from build123d import *

# Parameters (mm, degrees)
SKETCH1_W           = 40
SKETCH1_H           = 43
SKETCH1_R           = 1.5
SKETCH1_R_2         = 5
BOSS_EXTRUDE1_DEPTH = 3
SKETCH3_R           = 1.6
BOSS_EXTRUDE2_DEPTH = 3
FILLET1_R           = 2


with BuildPart() as part:
    # Sketch1 → Boss-Extrude1 (new body)
    with BuildSketch(Plane(origin=(0, 0, 0), x_dir=(1, 0, 0), z_dir=(0, 1, 0))):
        Rectangle(SKETCH1_W, SKETCH1_H)
        with Locations((-15, -11.5)):
            Circle(SKETCH1_R, mode=Mode.SUBTRACT)
        with Locations((15, -11.5)):
            Circle(SKETCH1_R, mode=Mode.SUBTRACT)
        with Locations((-15, 8.5)):
            Circle(SKETCH1_R, mode=Mode.SUBTRACT)
        with Locations((15, 8.5)):
            Circle(SKETCH1_R, mode=Mode.SUBTRACT)
        Circle(SKETCH1_R_2, mode=Mode.SUBTRACT)
    extrude(amount=BOSS_EXTRUDE1_DEPTH)

    # Sketch3 → Boss-Extrude2 (add)
    with BuildSketch(Plane(origin=(0, 0, -21.5), x_dir=(-1, 0, 0), z_dir=(0, 0, -1))):
        with BuildLine():
            Line((-20, 3), (20, 3))
            Line((20, 3), (20, 30))
            ThreePointArc((20, 30), (0, 50), (-20, 30))
            Line((-20, 30), (-20, 3))
        make_face()
        with Locations((0, 16)):
            Circle(SKETCH3_R, mode=Mode.SUBTRACT)
        with Locations((-9.899494937, 20.100505063)):
            Circle(SKETCH3_R, mode=Mode.SUBTRACT)
        with Locations((-14, 30)):
            Circle(SKETCH3_R, mode=Mode.SUBTRACT)
        with Locations((-9.899494937, 39.899494937)):
            Circle(SKETCH3_R, mode=Mode.SUBTRACT)
        with Locations((9.899494937, 39.899494937)):
            Circle(SKETCH3_R, mode=Mode.SUBTRACT)
        with Locations((14, 30)):
            Circle(SKETCH3_R, mode=Mode.SUBTRACT)
        with Locations((9.899494937, 20.100505063)):
            Circle(SKETCH3_R, mode=Mode.SUBTRACT)
        with BuildLine():
            ThreePointArc((-5.421047417, 39.571428571), (0, 19), (5.421047417, 39.571428571))
            ThreePointArc((5.421047417, 39.571428571), (3.680856516, 41.738279783), (1.15096765, 42.888571429))
            ThreePointArc((1.15096765, 42.888571429), (0, 45.6), (-1.15096765, 42.888571429))
            ThreePointArc((-1.15096765, 42.888571429), (-3.680856516, 41.738279783), (-5.421047417, 39.571428571))
        make_face(mode=Mode.SUBTRACT)
    extrude(amount=-BOSS_EXTRUDE2_DEPTH)

    # Fillet1
    fillet1_edges = [part.edges().sort_by_distance(p)[0] for p in [
        (0, 3, -18.5),
        (0, 0, -21.5),
        (20, 1.5, 21.5),
        (-20, 1.5, 21.5),
    ]]
    fillet(fillet1_edges, radius=FILLET1_R)


solid = part.part
Verification items for the finished model (mm, model axes). A direction names the side the tool comes from. Round coordinates to 2 decimals unless told otherwise and drop trailing zeros. Loops run counter-clockwise (first coordinate to the right, second up) from the corner with the lowest first, then second, coordinate; pieces in that order, holes last. Notation, with made-up numbers: (3, 31) - (29, 31) arc R13 cw to (29, 49) - close; hole circle Ø4 at (-27.5, 82). An arc over 180 degrees is marked (long way). Use one line per item in the form item = value.
1. Section check A-A on y = 16. Record the cut outline in (x, z).
A:
outline = (-20, -21.5) - (-1.6, -21.5) - (-1.6, -18.5) - (-20, -18.5) - close; (1.6, -21.5) - (20, -21.5) - (20, -18.5) - (1.6, -18.5) - close
2. Section check B-B on z = 4. Record the cut outline in (x, y), and give its area (3 significant figures).
A:
outline = (-20, 0) - (-3, 0) - (-3, 3) - (-20, 3) - close; (3, 0) - (20, 0) - (20, 3) - (3, 3) - close
area = 102 mm²
3. Gauge pin test, flat ends, axial feed: pin 1 Ø5 at (x, z) = (-15, 11.5) entering from +Y; pin 2 Ø3.5 at (x, y) = (-9.9, 20.1) entering from +Z; pin 3 Ø2.5 at (x, y) = (14, 30) entering from +Z. Record the tip position at first contact, or that the pin passes through.
A:
pin_1 = 3
pin_2 = -18.5
pin_3 = through
4. Draft check along Y on faces 3 (the flat face through (-0.3, 0, 5.3)), 4 (the cylindrical face through (-3.712, 41.714, -20.021)), 5 (the cylindrical face through (-16.5, 1.48, 11.43)). Enter one of: pulls with the +Y half, pulls with the -Y half, needs draft (parallel to the pull), parting line crosses it, or undercut.
A:
face_3 = pulls with the -Y half
face_4 = undercut
face_5 = needs draft
5. Scan lines: probe 1 along X at (y, z) = (2.3, -8.5); probe 2 along X at (y, z) = (1, -8); probe 3 along Z at (x, y) = (-18, 17). Record each from-to range of solid material in increasing order.
A:
probe_1 = -20 to -16.5, -13.5 to 13.5, 16.5 to 20
probe_2 = -20 to -16.41, -13.59 to 13.59, 16.41 to 20
probe_3 = -21.5 to -18.5
6. Access from +Z, -Z, +X, -X, +Y, -Y to the whole of each face (thin tool, end or side, straight path). Record for faces 1 (the cylindrical face through (3.6, 41.8, -20)), 2 (the flat face through (-4, 16, -21.5)).
A:
face_1 = +Z, -Z
face_2 = -Z, +X, -X, +Y, -Y
7. Section check C-C on z = -8.5. Record the cut outline in (x, y), and give its area (3 significant figures).
A:
outline = (-20, 0) - (-16.5, 0) - (-16.5, 3) - (-20, 3) - close; (-13.5, 0) - (13.5, 0) - (13.5, 3) - (-13.5, 3) - close; (16.5, 0) - (20, 0) - (20, 3) - (16.5, 3) - close
area = 102 mm²
8. Section check D-D on y = 11. Record the cut outline in (x, z), and give its area (3 significant figures).
A:
outline = (-20, -21.5) - (20, -21.5) - (20, -18.5) - (-20, -18.5) - close
area = 120 mm²
